Design review of the part shown in the three views and the two pictorial views. Dimensions are in mm from the part's minimum x, y and z. A direction names the side the tool comes from. Coordinates: 2 decimals unless noted, no trailing zeros. Loops run counter-clockwise (first coordinate to the right, second up) from the corner with the lowest first, then second, coordinate; pieces in that order, holes last. Notation, with made-up numbers: (-22, 71.5) -> (12, 71.5) arc R23 ccw to (12, 82.5) -> close; hole circle Ø10 at (6, -10). An arc over 180 degrees is marked (long way). One line per item, written item: value. Start each with the question number.
1. Add section B-B on z = 18. Write out the cut boundary in (x, y).
2. For probe 1 along Y at (x, z) = (3, 35.5); probe 2 along Z at (x, y) = (3.75, 17.5); probe 3 along Z at (x, y) = (2, 17.5), list the stretches that pass through material, from the lowest coordinate up.
3. Add section C-C on y = 26.5. Write out the cut boundary in (x, z).
4. Insertion check: pin 1 (1.5 mm diameter, centred on x = 14.5, y = 26, fed in from +Z); pin 2 (5 mm diameter, centred on x = 17.5, z = 22.5, fed in from +Y); pin 3 (8 mm diameter, centred on x = 5, y = 33, fed in from +Z). Each pin has a flat end and moves straight along its axis. Give the tip position at first contact, or say it passes through.
5. Machinability: for the marked faces 1 and 2, which of the approach directions +Z, -Z, +X, -X, +Y, -Y give a long, thin tool a straight path to every point of the face, cutting with its end or side? Answer none if there is none.
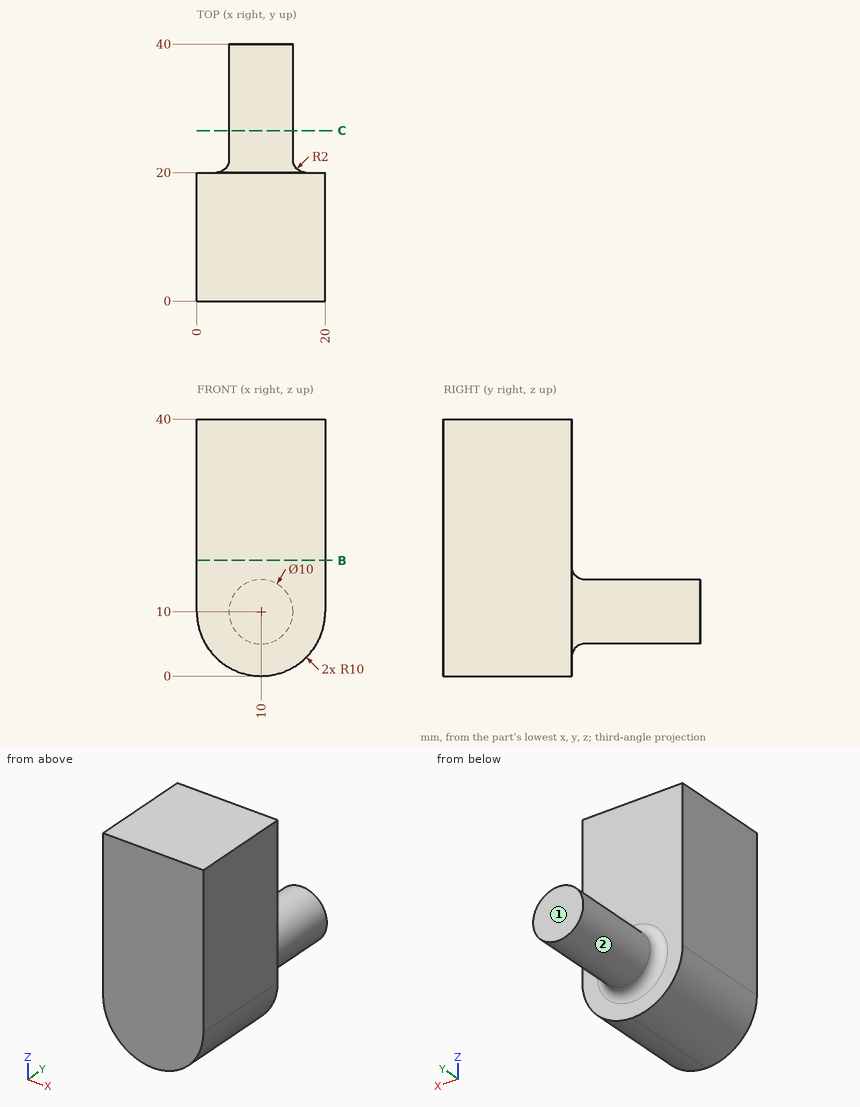
Worked answers:
1. outline: (0, 0) -> (20, 0) -> (20, 20) -> (0, 20) -> close
2. probe 1: y = 0 to 20
2. probe 2: z = 2.19 to 40
2. probe 3: z = 4 to 40
3. outline: circle Ø10 at (10, 10)
4. pin 1: stops at z = 13.31
4. pin 2: stops at y = 20
4. pin 3: stops at z = 14.9
5. face 1: +Z, -Z, +X, -X, +Y
5. face 2: +Y
